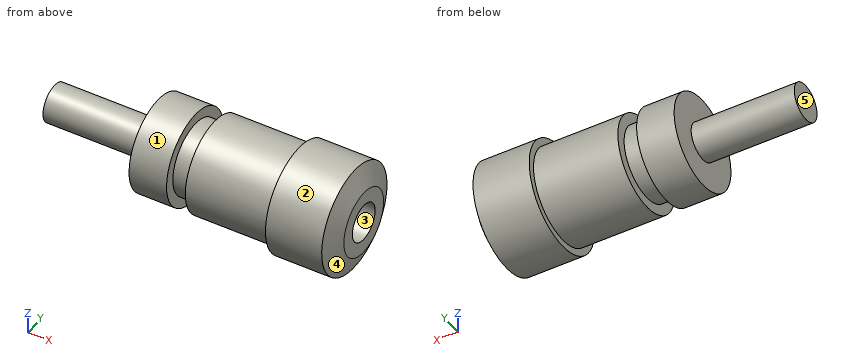
```python
from build123d import *


with BuildPart() as f1:
    # F0 (on Front) → F1 (revolve)
    with BuildSketch(Plane.XZ):
        Polygon((-17, 2), (-17, 0), (1, 0), (1, 2), (16, 2), (16, 3.5), (15, 5.75), (9, 5.75), (9, 5), (0, 5), (0, 3.9), (-2, 3.9), (-2, 2), (-6, 2), align=None)
        Polygon((-6, 5), (-6, 2), (-2, 2), (-2, 3.9), (-2, 5), align=None)
    revolve(axis=Axis((-8, 0, 0), (-1, 0, 0)))


solid = f1.part
```
CAD build for the part. Positions are in the model's coordinates, mm. Face numbers are marked on the shaded views. A direction names the side the tool comes from. Give positions to 0.01 mm unless a question says otherwise; leave off trailing zeros. Write each loop counter-clockwise with the first axis right and the second up, starting at its lowest first coordinate (ties: lowest second). Pieces come first, ordered by that corner, then holes. Notation, with made-up numbers: M 25,-28 L 45,-28 A26 cw 45,-1 Z; hole C -34.75,80 d4. An arc over 180 degrees is marked long. Return JSON: item names as keys, results as strings. Group by question number.
(1) Band-saw the part on D-D (x = -9). Give the cut face in (y, z), and give its area (3 significant figures).
(2) Drill centre lines: L1, parallel to Y at x = 5.5, z = 0; L2, parallel to Y at x = 10, z = 0; L3, parallel to Z at x = -3, y = 0.25. Where is each one in solid material? Low to high. Write a range as [from, to].
(3) 3-axis set-ups, long thin cutter, end or side, ignore diameter. For the marked faces 1 and 2: which of +Z, -Z, +X, -X, +Y, -Y reach the whole face in a straight line?
(4) Mould opens along Y. For the marked faces 3, 4 and 5 say: pulls with the +Y half, pulls with the -Y half, needs draft (parallel to the pull), parting line crosses it, or undercut.
(5) Band-saw the part on B-B (x = 14). Give the cut face in (y, z), and give its area (3 significant figures).
(6) Flat gauge pins, fed straight in: pin 1 Ø2 at (x, y) = (1, -2) entering from +Z; pin 2 Ø1.2 at (y, z) = (-0.5, 0) entering from +X; pin 3 Ø1.5 at (x, z) = (-8, 1) entering from +Y. Where does each tip first touch, or does it go through?
(7) Band-saw the part on A-A (y = 0). Give the cut face in (x, z), and give its area (3 significant figures).
Entries:
{
 "1": {"outline": "C 0,0 d4", "area": "12.6 mm^2"},
 "2": {"L1": "y = [-5, -2], [2, 5]", "L2": "y = [-5.75, -2], [2, 5.75]", "L3": "z = [-4.99, 4.99]"},
 "3": {"face 1": "-X", "face 2": "+X, -X"},
 "4": {"face 3": "undercut", "face 4": "parting line crosses it", "face 5": "needs draft"},
 "5": {"outline": "C 0,0 d11.5; hole C 0,0 d4", "area": "91.3 mm^2"},
 "6": {"pin 1": "stops at z = 4.9", "pin 2": "stops at x = 1", "pin 3": "stops at y = 1.98"},
 "7": {"outline": "M -17,-2 L -6,-2 L -6,-5 L -2,-5 L -2,-3.9 L 0,-3.9 L 0,-5 L 9,-5 L 9,-5.75 L 15,-5.75 L 16,-3.5 L 16,-2 L 1,-2 L 1,2 L 16,2 L 16,3.5 L 15,5.75 L 9,5.75 L 9,5 L 0,5 L 0,3.9 L -2,3.9 L -2,5 L -6,5 L -6,2 L -17,2 Z", "area": "208 mm^2"}
}
